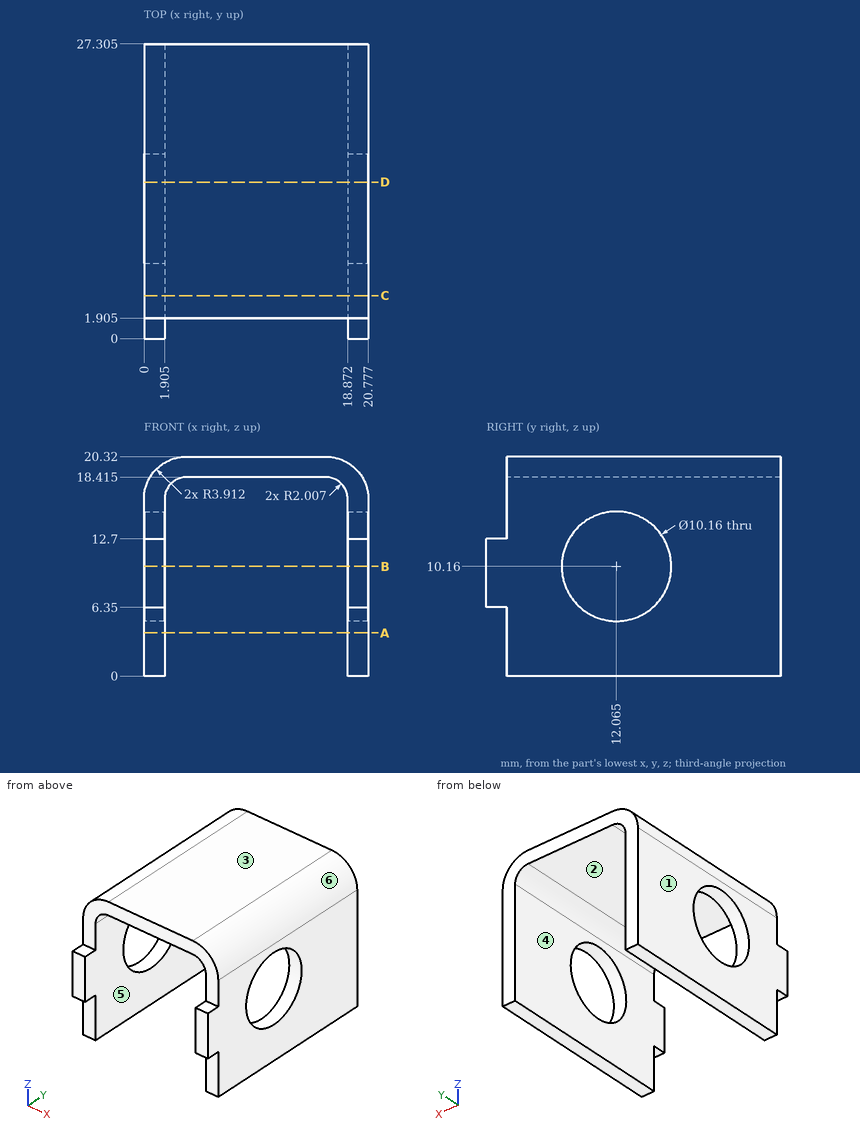
Verification items for this drawing (mm, ordinates from the low corner). A direction names the side the tool comes from. Coordinates: 2 decimals unless noted, no trailing zeros. Order: outer loops, then holes, each group sorted by start corner. A loop starts at its lowest first (then second) coordinate and runs counter-clockwise, first axis right, second up. Notation, with made-up numbers: M -25,79 L -13,79 A17 ccw -13,100 Z; hole C -22.75,-39 d4. An arc over 180 degrees is marked long. Write each question's results on one line, items separated by ' | '.
1) Gauge pin test, flat ends, axial feed: pin 1 Ø1.5 at (x, y) = (1, 1) entering from -Z; pin 2 Ø0.6 at (x, z) = (0.5, 3) entering from -Y (3 decimals); pin 3 Ø0.6 at (x, y) = (20, 1) entering from +Z. Record the tip position at first contact, or that the pin passes through.
Solved:
pin 1: stops at z = 6.35 | pin 2: stops at y = 1.905 | pin 3: stops at z = 12.7
2) Release check for a two-part mould opening along X. For the marked faces 1, 2, 3 and 4 record: pulls with the +X half, pulls with the -X half, needs draft (parallel to the pull), parting line crosses it, or undercut.
Solved:
face 1: pulls with the -X half | face 2: undercut | face 3: needs draft | face 4: undercut
3) Section check B-B on z = 10.16. Record the cut outline in (x, y) (1 decimal).
Solved:
outline: M 0,0 L 1.9,0 L 1.9,7 L 0,7 Z; M 0,17.1 L 1.9,17.1 L 1.9,27.3 L 0,27.3 Z; M 18.9,0 L 20.8,0 L 20.8,7 L 18.9,7 Z; M 18.9,17.1 L 20.8,17.1 L 20.8,27.3 L 18.9,27.3 Z
4) Section check C-C on y = 4. Record the cut outline in (x, z) (1 decimal), plus the area to 3 significant figures.
Solved:
outline: M 0,0 L 1.9,0 L 1.9,16.4 A2 cw 3.9,18.4 L 16.9,18.4 A2 cw 18.9,16.4 L 18.9,0 L 20.8,0 L 20.8,16.4 A3.9 ccw 16.9,20.3 L 3.9,20.3 A3.9 ccw 0,16.4 Z | area: 105 mm²
5) Section check A-A on z = 4. Record the cut outline in (x, y) (1 decimal).
Solved:
outline: M 0,1.9 L 1.9,1.9 L 1.9,27.3 L 0,27.3 Z; M 18.9,1.9 L 20.8,1.9 L 20.8,27.3 L 18.9,27.3 Z
6) Access from +Z, -Z, +X, -X, +Y, -Y to the whole of each face (thin tool, end or side, straight path). Record for the marked faces 5 and 6.
Solved:
face 5: -Z, +Y, -Y | face 6: +Z, +X, +Y, -Y
7) Section check D-D on y = 14.5. Record the cut outline in (x, z) (1 decimal).
Solved:
outline: M 0,0 L 1.9,0 L 1.9,5.7 L 0,5.7 Z; M 0,14.6 L 1.9,14.6 L 1.9,16.4 A2 cw 3.9,18.4 L 16.9,18.4 A2 cw 18.9,16.4 L 18.9,14.6 L 20.8,14.6 L 20.8,16.4 A3.9 ccw 16.9,20.3 L 3.9,20.3 A3.9 ccw 0,16.4 Z; M 18.9,0 L 20.8,0 L 20.8,5.7 L 18.9,5.7 Z
8) Scan lines: line 1 along X through (y, z) = (22, 16.25) (1 decimal); line 2 along Y through (x, z) = (1.25, 10.16) (1 decimal); line 3 along Z through (x, y) = (15.75, 20.25) (1 decimal). Record each from-to range of solid material in increasing order. Write a range as [from, to].
Solved:
line 1: x = [0, 1.9], [18.9, 20.8] | line 2: y = [0, 7], [17.1, 27.3] | line 3: z = [18.4, 20.3]
